```python
from build123d import *

# Parameters (mm, degrees)
SKETCH1_W           = 29.21
SKETCH1_H           = 30.226
BOSS_EXTRUDE1_DEPTH = 6.731
SKETCH2_W           = 5.1816
SKETCH2_H           = 2.1336
BOSS_EXTRUDE2_DEPTH = 13.462
SKETCH3_R           = 2.88925
BOSS_EXTRUDE3_DEPTH = 5.0038


with BuildPart() as part:
    # Sketch1 → Boss-Extrude1 (new body, symmetric)
    with BuildSketch(Plane.XY):
        Rectangle(SKETCH1_W, SKETCH1_H)
    extrude(amount=BOSS_EXTRUDE1_DEPTH, both=True)

    # Sketch2 → Boss-Extrude2 (add)
    with BuildSketch(Plane.XY.offset(6.731)):
        with Locations((-17.1958, 6.2357)):
            Rectangle(SKETCH2_W, SKETCH2_H)
    boss_extrude2 = extrude(amount=-BOSS_EXTRUDE2_DEPTH)

    # Mirror1: Boss-Extrude2 across plane
    add(boss_extrude2.mirror(Plane(origin=(0, 0, 0), x_dir=(0, 0, 1), z_dir=(1, 0, 0))))

    # Sketch3 → Boss-Extrude3 (add)
    with BuildSketch(Plane(origin=(0, 15.113, 0), x_dir=(1, 0, 0), z_dir=(0, 1, 0))):
        with Locations((8.64235, 0)):
            Circle(SKETCH3_R)
    extrude(amount=BOSS_EXTRUDE3_DEPTH)


solid = part.part
```
Check sheet for the modelled part. Datum: model origin and axes. Units: mm. A direction names the side the tool comes from. Round coordinates to 2 decimals unless told otherwise and drop trailing zeros. Write each loop counter-clockwise with the first axis right and the second up, starting at its lowest first coordinate (ties: lowest second). Pieces come first, ordered by that corner, then holes. Notation, with made-up numbers: (28.5, -12) -> (41.5, -12) arc R5 cw to (41.5, -5) -> close; hole circle Ø2 at (-34.75, -19.75). An arc over 180 degrees is marked (long way). One line per question, with ' | ' between items. Start each with the question number.
1. Scan lines: line 1 along X through (y, z) = (0.5, 3) (3 decimals); line 2 along Y through (x, z) = (16.5, 5); line 3 along Y through (x, z) = (7, 6). Record each from-to range of solid material in increasing order. Write a range as from..to.
2. Sectioned sample at B-B, the plane x = 7. Record the cut outline in (y, z), then the cut area to 3 significant figures.
3. Depth check by flat-ended pin: pin 1 (2.5 mm diameter, centred on y = 9.5, z = -2.5, fed in from +X) (3 decimals); pin 2 (2.5 mm diameter, centred on x = 17.5, z = 1.5, fed in from +Y); pin 3 (1 mm diameter, centred on y = -6, z = -1, fed in from -X) (3 decimals). Enter the tip coordinate at first touch or a pass-through.
4. Sectioned sample at A-A, the plane z = 0. Record the cut outline in (x, y) (1 decimal).
5. Set-up check for faces 1 (the face through (-14.605, 11, 0)), 2 (the face through (17, 5.169, 0)), 3 (the face through (17, 7.302, 0)), 4 (the face through (10.196, 17.58, -2.436)): record each of +Z, -Z, +X, -X, +Y, -Y from which the full face is reachable in a straight line by a thin tool's end or side.
6. Sectioned sample at C-C, the plane y = 14. Record the cut outline in (x, z) (3 decimals), then the cut area to 3 significant figures.
7. Sectioned sample at D-D, the plane x = 13. Record the cut outline in (y, z).
Taken from the geometry:
1) line 1: x = -14.605..14.605 | line 2: y = 5.17..7.3 | line 3: y = -15.11..15.11
2) outline: (-15.11, -6.73) -> (15.11, -6.73) -> (15.11, -2.38) -> (20.12, -2.38) -> (20.12, 2.38) -> (15.11, 2.38) -> (15.11, 6.73) -> (-15.11, 6.73) -> close | area: 431 mm^2
3) pin 1: stops at x = 14.605 | pin 2: stops at y = 7.3 | pin 3: stops at x = -14.605
4) outline: (-19.8, 5.2) -> (-14.6, 5.2) -> (-14.6, -15.1) -> (14.6, -15.1) -> (14.6, 5.2) -> (19.8, 5.2) -> (19.8, 7.3) -> (14.6, 7.3) -> (14.6, 15.1) -> (11.5, 15.1) -> (11.5, 20.1) -> (5.8, 20.1) -> (5.8, 15.1) -> (-14.6, 15.1) -> (-14.6, 7.3) -> (-19.8, 7.3) -> close
5) face 1: +Z, -Z, -X, +Y | face 2: +Z, -Z, +X, -Y | face 3: +Z, -Z, +X, +Y | face 4: +Y
6) outline: (-14.605, -6.731) -> (14.605, -6.731) -> (14.605, 6.731) -> (-14.605, 6.731) -> close | area: 393 mm^2
7) outline: (-15.11, -6.73) -> (15.11, -6.73) -> (15.11, 6.73) -> (-15.11, 6.73) -> close
